```python
from build123d import *

# Parameters (mm, degrees)
ESQUISSE1_R          = 3.5
BASE_EXTRUSION_DEPTH = 40
ESQUISSE2_R          = 2
BOSS_EXTRU_1_DEPTH   = 61.3
ESQUISSE3_R          = 1.55
BOSS_EXTRU_2_DEPTH   = 0.7
ESQUISSE4_R          = 2
BOSS_EXTRU_3_DEPTH   = 2
CONG_1_R             = 0.5
PER_AGE1_D           = 1.5
PER_AGE1_DEPTH       = 11
PER_AGE1_CBORE_D     = 3
PER_AGE1_CBORE_DEPTH = 8
PER_AGE1_TIP         = 0.433012702


with BuildPart() as part:
    # Esquisse1 → Base-Extrusion (new body)
    with BuildSketch(Plane.XY):
        Circle(ESQUISSE1_R)
    extrude(amount=BASE_EXTRUSION_DEPTH)

    # Esquisse2 → Boss.-Extru.1 (add)
    with BuildSketch(Plane(origin=(0, 0, 0), x_dir=(-1, 0, 0), z_dir=(0, 0, -1))):
        Circle(ESQUISSE2_R)
    extrude(amount=-BOSS_EXTRU_1_DEPTH)

    # Esquisse3 → Boss.-Extru.2 (add)
    with BuildSketch(Plane.XY.offset(61.3)):
        Circle(ESQUISSE3_R)
    extrude(amount=BOSS_EXTRU_2_DEPTH)

    # Esquisse4 → Boss.-Extru.3 (add)
    with BuildSketch(Plane.XY.offset(62)):
        with Locations(Location((0, 0, 0), (0, 0, 180))):
            Circle(ESQUISSE4_R)
    extrude(amount=BOSS_EXTRU_3_DEPTH)

    # Congé1
    cong_1_edges = [part.edges().sort_by_distance(p)[0] for p in [
        (2, 0, 40),
    ]]
    fillet(cong_1_edges, radius=CONG_1_R)

    # Perçage1
    with Locations(Plane(origin=(0, 0, 0), x_dir=(-1, 0, 0), z_dir=(0, 0, -1))):
        with Locations((0, 0)):
            CounterBoreHole(PER_AGE1_D / 2, PER_AGE1_CBORE_D / 2, PER_AGE1_CBORE_DEPTH, depth=PER_AGE1_DEPTH)
            with Locations((0, 0, -(PER_AGE1_DEPTH + PER_AGE1_TIP / 2))):  # 120° drill point
                Cone(0, PER_AGE1_D / 2, PER_AGE1_TIP, mode=Mode.SUBTRACT)


solid = part.part
```
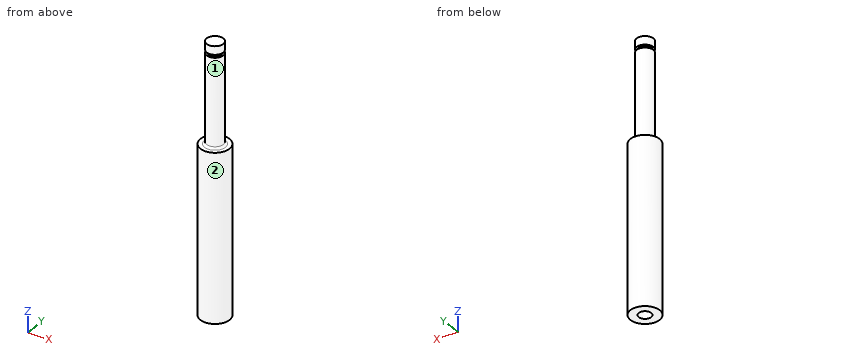
The model under review builds one solid part; all positions refer to its coordinate system, in mm. Face numbers are marked on the shaded views. A direction names the side the tool comes from. Round coordinates to 2 decimals unless told otherwise and drop trailing zeros. Loops run counter-clockwise (first coordinate to the right, second up) from the corner with the lowest first, then second, coordinate; pieces in that order, holes last. Notation, with made-up numbers: (-31.75, 65.25) - (7.25, 65.25) arc R21 ccw to (7.25, 93.25) - close; hole circle Ø6 at (4.25, -25.75). An arc over 180 degrees is marked (long way). Use a Markdown table: item, result. Add a question column.
Q1. Insertion check: pin 1 Ø1 at (y, z) = (1, 24) entering from -X; pin 2 Ø1.4 at (x, y) = (0, 0) entering from -Z; pin 3 Ø3 at (x, z) = (0.5, 54) entering from -Y. Each pin has a flat end and moves straight along its axis. Give the tip position at first contact, or say it passes through.
Q2. For probe 1 along Z at (x, y) = (-0.75, -1.5); probe 2 along Y at (x, z) = (0, 1.75); probe 3 along Y at (x, z) = (0, 10), list the stretches that pass through material, from the lowest coordinate up.
Q3. Add section A-A (z = 5). State the section outline as (x, y) points, plus the area to 3 significant figures.
Q4. Machinability: for the marked faces 1 and 2, which of the approach directions +Z, -Z, +X, -X, +Y, -Y give a long, thin tool a straight path to every point of the face, cutting with its end or side? Answer none if there is none.
Q5. Add section B-B (z = 39). State the section outline as (x, y) points, plus the area to 3 significant figures.
Worked answers:
| question | item | result |
|---|---|---|
| 1 | pin 1 | x = -3.46 |
| 1 | pin 2 | z = 11.03 |
| 1 | pin 3 | y = -2 |
| 2 | probe 1 | 0 to 61.3, 62 to 64 |
| 2 | probe 2 | -3.5 to -1.5, 1.5 to 3.5 |
| 2 | probe 3 | -3.5 to -0.75, 0.75 to 3.5 |
| 3 | outline | circle Ø7 at (0, 0); hole circle Ø3 at (0, 0) |
| 3 | area | 31.4 mm² |
| 4 | face 1 | +Z |
| 4 | face 2 | +Z, -Z |
| 5 | outline | circle Ø7 at (0, 0) |
| 5 | area | 38.5 mm² |
